The model under review builds one solid part; all positions refer to its coordinate system, in mm. A direction names the side the tool comes from. Coordinates: 2 decimals unless noted, no trailing zeros. Order: outer loops, then holes, each group sorted by start corner. A loop starts at its lowest first (then second) coordinate and runs counter-clockwise, first axis right, second up. Notation, with made-up numbers: (55, 48.25) -> (62, 48.25) arc R37 ccw to (62, 86.25) -> close; hole circle Ø9 at (67, 41.5). An arc over 180 degrees is marked (long way). Use one line per item in the form item = value.
Autodesk Inventor part; units mm, degrees
ref_plane "YZ Plane" through (0, 0, 0) normal (1, 0, 0) x (0, 1, 0)
ref_plane "XZ Plane" through (0, 0, 0) normal (0, 1, 0) x (-1, 0, 0)
ref_plane "XY Plane" through (0, 0, 0) normal (0, 0, 1) x (1, 0, 0)
sketch "Sketch1" plane through (0, 0, 0) normal (0, 0, 1) x (1, 0, 0)
  line L0 (-11.5, 11) -> (11.5, 11)
  line L1 (11.5, 11) -> (11.5, -11)
  line L2 (11.5, -11) -> (-11.5, -11)
  line L3 (-11.5, -11) -> (-11.5, 11)
  line L4 (-11.5, 11) -> (11.5, -11) construction
  line L5 (11.5, 11) -> (-11.5, -11) construction
  point P0 (0, 0)
  dimension "d0" = 23
  dimension "d1" = 22
extrude "Extrusion1" add sketch "Sketch1" along normal blind 3
sketch "Sketch2" plane through (0, 0, 3) normal (0, 0, 1) x (1, 0, 0)
  line L0 (11.5, 11) -> (-11.5, 11)
  line L1 (-11.5, 11) -> (-15, 11)
  line L2 (-15, 11) -> (-15, -11)
  line L3 (-15, -11) -> (-11.5, -11)
  line L4 (-11.5, -11) -> (-11.5, 11)
  line L5 (-11.5, -11) -> (11.5, -11)
  line L6 (11.5, -11) -> (15, -11)
  line L7 (15, -11) -> (15, 11)
  line L8 (15, 11) -> (11.5, 11)
  line L9 (11.5, 11) -> (11.5, -11)
  point P0 (0, 0)
  dimension "d4" = 3.5
  dimension "d5" = 3.5
extrude "Extrusion2" add sketch "Sketch2" against normal blind 8.5 contours L8 L7 L6 L9 | L4 L3 L2 L1
sketch "Sketch3" plane through (15, -11, 3) normal (1, 0, 0) x (0, 0, -1)
  line L0 (0, 0) -> (0, 22) construction
  line L1 (0, 22) -> (8.5, 22) construction
  line L2 (8.5, 22) -> (8.5, 0) construction
  line L3 (8.5, 0) -> (0, 0) construction
  circle A0 centre (5, 19) radius 1
  circle A1 centre (5, 3) radius 1
  line L4 (3, 22) -> (3, 0) construction
  arc A2 (5, 16) -> (5, 22) centre (5, 19) ccw
  line L5 (5, 22) -> (5, 0) construction
  arc A3 (5, 0) -> (5, 6) centre (5, 3) ccw
  line L6 (5, 16) -> (5, 6)
  line L7 (3, 22) -> (8.5, 22)
  line L8 (5, 0) -> (8.5, 0)
  line L9 (8.5, 0) -> (8.5, 22)
  line L10 (8.5, 22) -> (5, 22)
  point P0 (3, 11)
  point P1 (3, 11)
  dimension "d8" = 2
  dimension "d9" = 2
  dimension "d10" = 16
  dimension "d11" = 2
  dimension "d12" = 8
extrude "Extrusion3" cut sketch "Sketch3" against normal through all
sketch "Sketch4" plane through (15, -11, 3) normal (1, 0, 0) x (0, 0, -1)
  line L0 (0, 0) -> (0, 22)
  line L1 (0, 21.5) -> (5, 21.5)
  line L2 (5, 21.5) -> (5, 23.5)
  line L3 (5, 23.5) -> (0, 23.5)
  line L4 (0, 23.5) -> (0, 21.5)
  line L5 (0, 22) -> (5, 22)
  line L6 (0, 0.5) -> (5, 0.5)
  line L7 (5, 0.5) -> (5, -1.5)
  line L8 (5, -1.5) -> (0, -1.5)
  line L9 (0, -1.5) -> (0, 0.5)
  line L10 (0, 0) -> (5, 0)
  dimension "d21" = 5
  dimension "d22" = 2
  dimension "d23" = 0.5
  dimension "d24" = 5
  dimension "d25" = 2
  dimension "d26" = 0.5
extrude "Extrusion4" [suppressed]
properties part number "Motor_Base"
Item 1: We need section D-D (x = -4.75). Write out the cut boundary in (y, z).
Results found:
outline = (-11, 0) -> (11, 0) -> (11, 3) -> (-11, 3) -> close
Item 2: We need section B-B (z = -4.5). Write out the cut boundary in (x, y).
Results found:
outline = (-15, -9.66) -> (-11.5, -9.66) -> (-11.5, -6.34) -> (-15, -6.34) -> close; (-15, 6.34) -> (-11.5, 6.34) -> (-11.5, 9.66) -> (-15, 9.66) -> close; (11.5, -9.66) -> (15, -9.66) -> (15, -6.34) -> (11.5, -6.34) -> close; (11.5, 6.34) -> (15, 6.34) -> (15, 9.66) -> (11.5, 9.66) -> close
Item 3: Draft analysis for pull direction Z (two halves, no side actions). For faces 4 (the face through (11.5, 0, -1)), 5 (the face through (-13, -7, -2)), 6 (the face through (13, 0, -2)), 7 (the face through (0, 0, 3)), state which applies: released by +Z, released by -Z, zero draft, split by the parting line, or undercut.
Results found:
face_4 = zero draft
face_5 = undercut
face_6 = released by -Z
face_7 = released by +Z
Item 4: We need section A-A (y = 8). Write out the cut boundary in (x, z).
Results found:
outline = (-15, -5) -> (-11.5, -5) -> (-11.5, -3) -> (-15, -3) -> close; (-15, -1) -> (-11.5, -1) -> (-11.5, 0) -> (11.5, 0) -> (11.5, -1) -> (15, -1) -> (15, 3) -> (-15, 3) -> close; (11.5, -5) -> (15, -5) -> (15, -3) -> (11.5, -3) -> close
Item 5: Tool access review of faces 1 (the face through (-13, 0, -2)), 2 (the face through (-13, 9, -2)), 3 (the face through (0, 0, 0)): name each direction out of +Z, -Z, +X, -X, +Y, -Y from which nothing blocks a thin tool from reaching the whole face with its end or side.
Results found:
face_1 = -Z, +X, -X
face_2 = +X, -X
face_3 = -Z, +Y, -Y
Item 6: Clearance check with flat-ended pins moving along their axes: pin 1 (1.2 mm diameter, centred on y = 8, z = -2, fed in from +X); pin 2 (3 mm diameter, centred on x = 14, y = -2, fed in from -Z); pin 3 (11 mm diameter, centred on x = 1, y = -4, fed in from -Z). State where each tip first meets the part, or that it passes through.
Results found:
pin_1 = through
pin_2 = -2
pin_3 = 0
Item 7: To check wall thickness, follow L1, parallel to X at y = -10, z = -3.5; L2, parallel to Z at x = -9.25, y = 0.5; L3, parallel to Z at x = 12.25, y = -6. State the ranges of each line that lie inside material, in increasing order. Write a range as from..to.
Results found:
L1 = -15..-11.5, 11.5..15
L2 = 0..3
L3 = -4.24..3
Item 8: We need section C-C (y = -2.5). Write out the cut boundary in (x, z), plus the area to 3 significant figures.
Results found:
outline = (-15, -2) -> (-11.5, -2) -> (-11.5, 0) -> (11.5, 0) -> (11.5, -2) -> (15, -2) -> (15, 3) -> (-15, 3) -> close
area = 104 mm²
